Geometry: see drawing. Coordinates: mm, zero at the bounding-box minimum. A direction names the side the tool comes from. Coordinates: 2 decimals unless noted, no trailing zeros. Order: outer loops, then holes, each group sorted by start corner. A loop starts at its lowest first (then second) coordinate and runs counter-clockwise, first axis right, second up.
Item 1: Section D-D on x = 8. Return the cut outline in (y, z), then the cut area to 3 significant figures.
Item 2: Mould query, pull axis Y, two halves, no side actions, for the marked faces 1, 2, 3 and 4. Classes: released by +Y, released by -Y, zero draft, split by the parting line, or undercut.
Item 3: Section A-A on x = 14.5. Return the cut outline in (y, z), then the cut area to 3 significant figures.
Item 4: Ray query, line 1 (Y direction, x = 27.5, z = 42); line 2 (Z direction, x = 12.5, y = 8.5); line 3 (X direction, y = 39, z = 18) (1 decimal). Return the intervals inside material, ascending.
Item 5: Section C-C on z = 6.5. Return the cut outline in (x, y) (1 decimal).
Item 6: Contact query for flat-ended pins moving along their axis: P1, Ø8, axis at x = 28.5, z = 49, coming from the +Y side; P2, Ø2, axis at x = 7.5, y = 25, coming from the +Z side; P3, Ø6, axis at x = 24.5, y = 21.5, coming from the +Z side; P4, Ø2, axis at y = 24.5, z = 26.5, coming from the -X side. Output: stop coordinate, or through.
Item 7: Reachability of the marked faces 5 and 6 from +Z, -Z, +X, -X, +Y, -Y: full face, straight path, thin tool, end or side. Return the list, or none.
Item 8: Section B-B on y = 23. Return the cut outline in (x, z) (1 decimal), then the cut area to 3 significant figures.
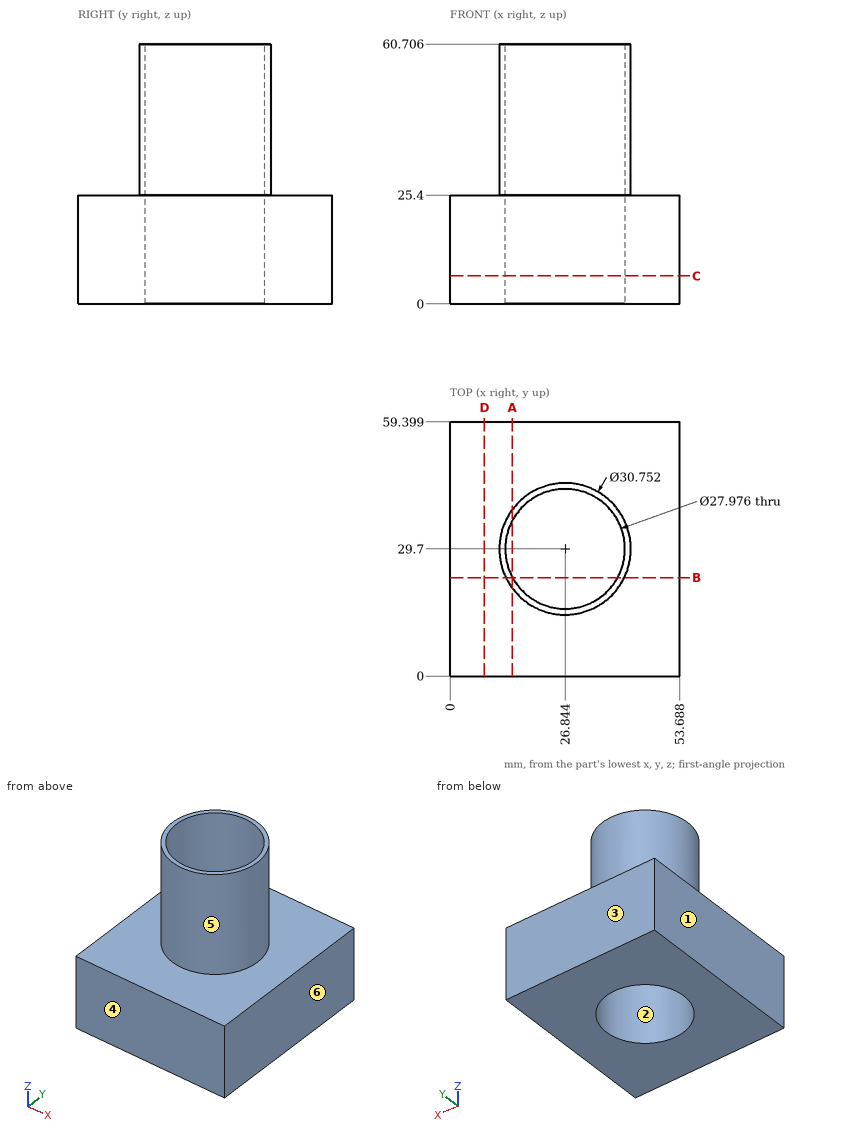
Answer list:
1. outline: (0, 0) - (59.4, 0) - (59.4, 25.4) - (0, 25.4) - close
1. area: 1,510 mm2
2. face 1: zero draft
2. face 2: undercut
2. face 3: released by +Y
2. face 4: released by -Y
3. outline: (0, 0) - (23.12, 0) - (23.12, 60.71) - (20.53, 60.71) - (20.53, 25.4) - (0, 25.4) - close; (36.28, 0) - (59.4, 0) - (59.4, 25.4) - (38.87, 25.4) - (38.87, 60.71) - (36.28, 60.71) - close
3. area: 1,360 mm2
4. line 1: y = 14.34 to 15.73, 43.67 to 45.06
4. line 2: z = 0 to 25.4
4. line 3: x = 0 to 16.4, 37.3 to 53.7
5. outline: (0, 0) - (53.7, 0) - (53.7, 59.4) - (0, 59.4) - close; hole circle Ø28 at (26.8, 29.7)
6. P1: stops at y = 45.08
6. P2: stops at z = 25.4
6. P3: passes through
6. P4: stops at x = 12.05
7. face 5: +Z
7. face 6: +Z, -Z, +X, +Y, -Y
8. outline: (0, 0) - (14.6, 0) - (14.6, 60.7) - (13, 60.7) - (13, 25.4) - (0, 25.4) - close; (39.1, 0) - (53.7, 0) - (53.7, 25.4) - (40.7, 25.4) - (40.7, 60.7) - (39.1, 60.7) - close
8. area: 850 mm2
